The model under review builds one solid part; all positions refer to its coordinate system, in mm. Give positions to 0.01 mm unless a question says otherwise; leave off trailing zeros. Order: outer loops, then holes, each group sorted by start corner. A loop starts at its lowest first (then second) coordinate and runs counter-clockwise, first axis right, second up. Notation, with made-up numbers: (83, -25) - (134, -25) arc R28 cw to (134, 6) - close; hole circle Ø10 at (37.5, 75). An arc over 180 degrees is marked (long way). Answer as CSV lines item,"result". Start each with the question number.
from build123d import *

# Parameters (mm, degrees)
SKETCH1_R           = 110
BOSS_EXTRUDE1_DEPTH = 22
SKETCH2_R           = 60
BOSS_EXTRUDE2_DEPTH = 120
SKETCH3_R           = 50
CUT_EXTRUDE1_DEPTH  = 211.627633515
SKETCH4_R           = 11.623448081
CUT_EXTRUDE2_DEPTH  = 197.468827044
FILLET1_R           = 3


with BuildPart() as part:
    # Sketch1 → Boss-Extrude1 (new body)
    with BuildSketch(Plane.XY):
        Circle(SKETCH1_R)
    extrude(amount=BOSS_EXTRUDE1_DEPTH)

    # Sketch2 → Boss-Extrude2 (add)
    with BuildSketch(Plane.XY.offset(22)):
        Circle(SKETCH2_R)
    extrude(amount=BOSS_EXTRUDE2_DEPTH)

    # Sketch3 → Cut-Extrude1 (cut, through all)
    with BuildSketch(Plane.XY.offset(142)):
        Circle(SKETCH3_R)
    extrude(amount=-CUT_EXTRUDE1_DEPTH, mode=Mode.SUBTRACT)

    # Sketch4 → Cut-Extrude2 (cut, through all)
    with BuildSketch(Plane.XY.offset(22)):
        with Locations((0, 85)):
            Circle(SKETCH4_R)
        with Locations((73.612159322, 42.5)):
            Circle(SKETCH4_R)
        with Locations((73.612159322, -42.5)):
            Circle(SKETCH4_R)
        with Locations((0, -85)):
            Circle(SKETCH4_R)
        with Locations((-73.612159322, -42.5)):
            Circle(SKETCH4_R)
        with Locations((-73.612159322, 42.5)):
            Circle(SKETCH4_R)
    extrude(amount=-CUT_EXTRUDE2_DEPTH, mode=Mode.SUBTRACT)

    # Fillet1
    fillet1_edges = [part.edges().sort_by_distance(p)[0] for p in [
        (-60, 0, 22),
    ]]
    fillet(fillet1_edges, radius=FILLET1_R)


solid = part.part
Item 1: Take a section at A-A on x = 0. Write out the cut boundary in (y, z).
Item 2: Take a section at D-D on y = -42.5. Count the separate pieces of the cut face and the enclosed holes in it, and give its area (3 significant figures).
Item 3: Clearance check with flat-ended pins moving along their axes: pin 1 (1 mm diameter, centred on x = 42.5, z = 94.5, fed in from -Y); pin 2 (6 mm diameter, centred on x = 83, y = 12.5, fed in from +Z); pin 3 (6 mm diameter, centred on x = -41, z = 64.5, fed in from -Y). State where each tip first meets the part, or that it passes through.
Item 4: For line 1 along Y through (x, z) = (0, 9); line 2 along X through (y, z) = (-1.5, 118.5); line 3 along X through (y, z) = (-42, 10), list the stretches that pass through material, from the lowest coordinate up.
Item 5: Take a section at B-B on z = 97.5. Write out the cut boundary in (x, y), and give its area (3 significant figures).
Item 6: Take a section at C-C on y = 85. Write out the cut boundary in (x, z).
Item 7: Mouldability with a two-part tool opening along Y and no side actions: class faces 1 (the face through (47, -47, 22)), 2 (the face through (-59.94, 2.64, 82.68)), 3 (the face through (6.25, 94.8, 11.15)), 4 (the face through (64.388, -49.573, 11.154)) as released by +Y, released by -Y, zero draft, split by the parting line, or undercut.
Data:
1,outline,"(-110, 0) - (-96.62, 0) - (-96.62, 22) - (-110, 22) - close; (-73.38, 0) - (-50, 0) - (-50, 142) - (-60, 142) - (-60, 25) arc R3 cw to (-63, 22) - (-73.38, 22) - close; (50, 0) - (73.38, 0) - (73.38, 22) - (63, 22) arc R3 cw to (60, 25) - (60, 142) - (50, 142) - close; (96.62, 0) - (110, 0) - (110, 22) - (96.62, 22) - close"
2,separate pieces,"4"
2,enclosed holes,"0"
2,area,"6,130 mm^2"
3,pin 1,"stops at y = -42.85"
3,pin 2,"stops at z = 22"
3,pin 3,"stops at y = -46.43"
4,line 1,"y = -110 to -96.62, -73.38 to -50, 50 to 73.38, 96.62 to 110"
4,line 2,"x = -59.98 to -49.98, 49.98 to 59.98"
4,line 3,"x = -101.67 to -85.22, -62 to -27.13, 27.13 to 62, 85.22 to 101.67"
5,outline,"circle Ø120 at (0, 0); hole circle Ø100 at (0, 0)"
5,area,"3,460 mm^2"
6,outline,"(-69.82, 0) - (-11.62, 0) - (-11.62, 22) - (-69.82, 22) - close; (11.62, 0) - (69.82, 0) - (69.82, 22) - (11.62, 22) - close"
7,face 1,"zero draft"
7,face 2,"split by the parting line"
7,face 3,"undercut"
7,face 4,"undercut"
